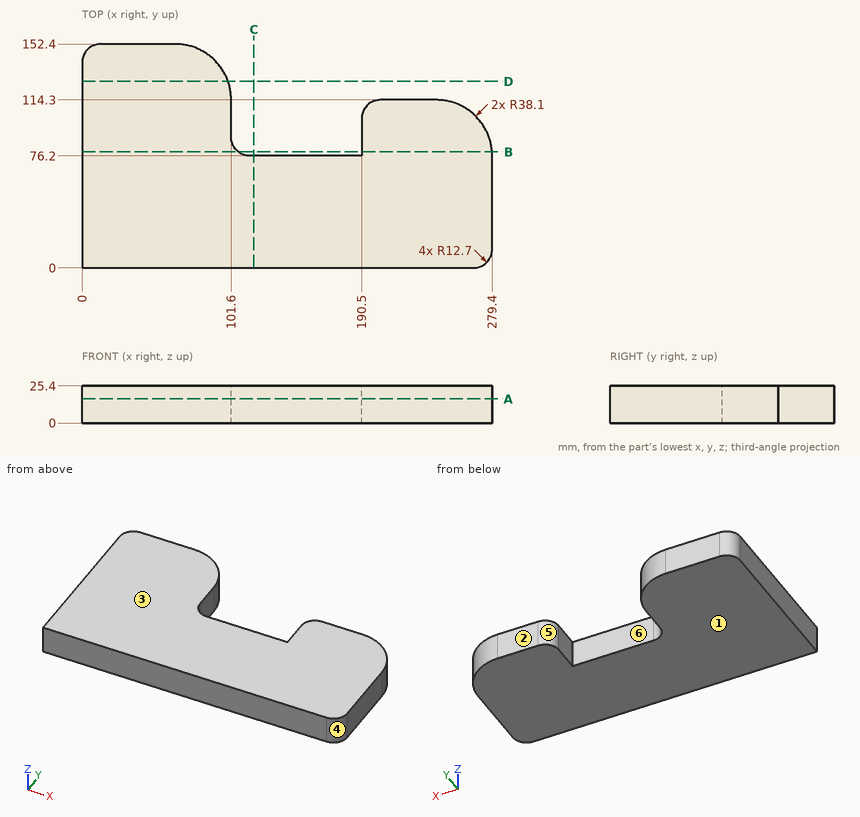
Here's the drawing with two shaded views (mm, measured from the low corner). I have some questions. A direction names the side the tool comes from. Give positions to 0.01 mm unless a question says otherwise; leave off trailing zeros. Order: outer loops, then holes, each group sorted by start corner. A loop starts at its lowest first (then second) coordinate and runs counter-clockwise, first axis right, second up. Notation, with made-up numbers: M 79,2 L 103,2 A25 ccw 103,15 Z; hole C 32,22.25 d10. An arc over 180 degrees is marked long. One line per item, written item: value.
1) On a 3-axis mill with a long thin cutter (end or side, diameter ignored), from which of +Z, -Z, +X, -X, +Y, -Y can I reach the whole of each face in a straight line? I mean the marked faces 1 and 2. Say none if no direction works.
Answer sheet:
face 1: -Z, +X, -X, +Y, -Y
face 2: +Z, -Z, +X, +Y
2) For P1, Ø12, axis at x = 210.5, y = 21.5, coming from the -Z side; P2, Ø7.5, axis at y = 105, z = 12.5, coming from the +X side; P3, Ø3, axis at y = 135.5, z = 17.5, coming from the +X side; P4, Ø7.5, axis at x = 228, z = 16.5, coming from the +Y side, each with a flat end and sliding along its axis, tell me the tip position at first contact or that it passes through.
Answer sheet:
P1: stops at z = 0
P2: stops at x = 270.01
P3: stops at x = 96.11
P4: stops at y = 114.3
3) I want a section at C-C, the plane x = 117. List the corners of the cut face in (y, z) for me.
Answer sheet:
outline: M 0,0 L 76.2,0 L 76.2,25.4 L 0,25.4 Z
4) I want a section at D-D, the plane y = 127. List the corners of the cut face in (x, z) for me.
Answer sheet:
outline: M 0,0 L 99.42,0 L 99.42,25.4 L 0,25.4 Z
5) I want a section at A-A, the plane z = 16.5. List the corners of the cut face in (x, y) for me, plus the area to 3 significant figures.
Answer sheet:
outline: M 0,0 L 266.7,0 A12.7 ccw 279.4,12.7 L 279.4,76.2 A38.1 ccw 241.3,114.3 L 203.2,114.3 A12.7 ccw 190.5,101.6 L 190.5,76.2 L 114.3,76.2 A12.7 cw 101.6,88.9 L 101.6,114.3 A38.1 ccw 63.5,152.4 L 12.7,152.4 A12.7 ccw 0,139.7 Z
area: 31,700 mm^2
6) Please list where these lines run through material, in increasing order: line 1 along Y through (x, z) = (212, 15); line 2 along X through (y, z) = (103.5, 23.75); line 3 along X through (y, z) = (101, 16).
Answer sheet:
line 1: y = 0 to 114.3
line 2: x = 0 to 101.6, 190.64 to 267.88
line 3: x = 0 to 101.6, 190.5 to 270.22
7) I want a section at B-B, the plane y = 79. List the corners of the cut face in (x, z) for me, plus the area to 3 significant figures.
Answer sheet:
outline: M 0,0 L 106.35,0 L 106.35,25.4 L 0,25.4 Z; M 190.5,0 L 279.3,0 L 279.3,25.4 L 190.5,25.4 Z
area: 4,960 mm^2
8) We'd pull the mould along X, two halves only. Please class the marked faces 3, 4, 5 and 6: released by +X, released by -X, zero draft, split by the parting line, or undercut.
Answer sheet:
face 3: zero draft
face 4: released by +X
face 5: undercut
face 6: undercut
